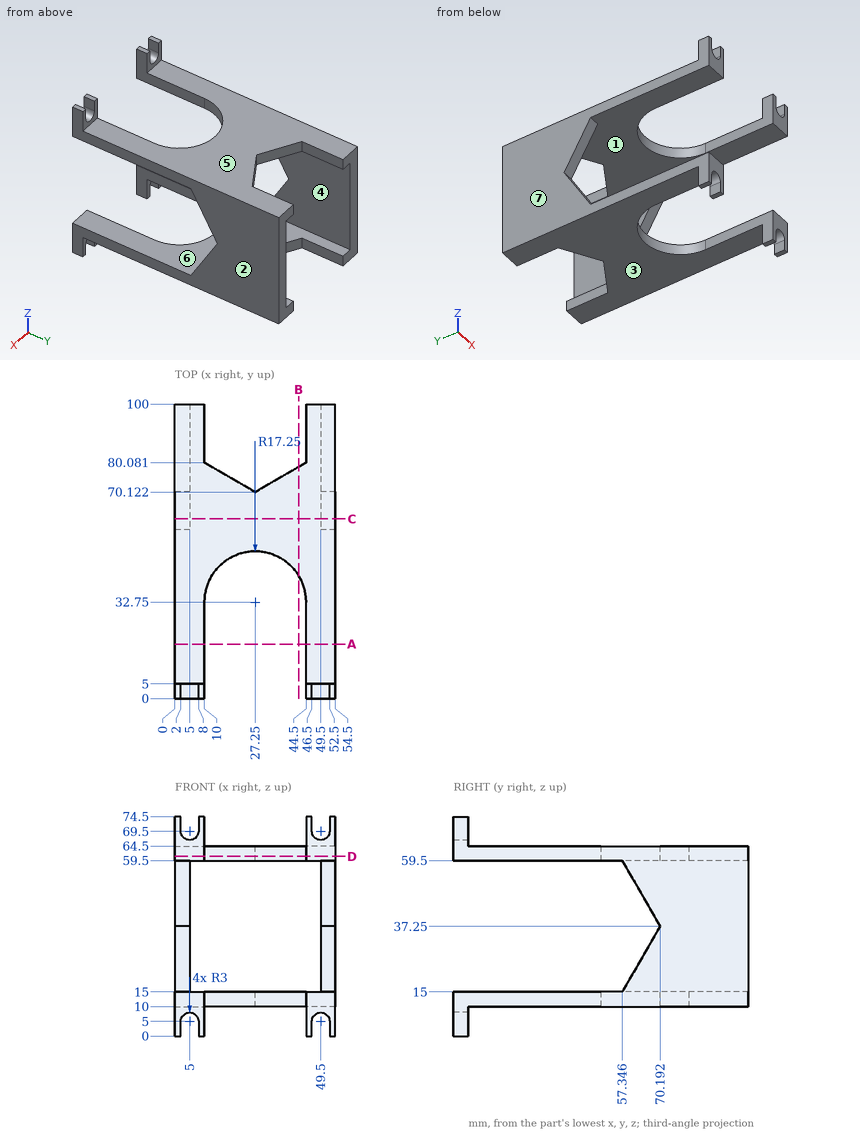
Input: dimensioned drawing with shaded views. Units: mm. Origin: part minimum x, y, z. A direction names the side the tool comes from. Coordinates: 2 decimals unless noted, no trailing zeros. Loops run counter-clockwise (first coordinate to the right, second up) from the corner with the lowest first, then second, coordinate; pieces in that order, holes last. Notation, with made-up numbers: M 39.5,-9 L 85.5,-9 A21 cw 85.5,27 Z; hole C 18,27 d4. An arc over 180 degrees is marked long. Put each result on its own line as item: value.
(1) Cut plane B-B on x = 42. Return the cut outline in (y, z) (1 decimal).
Answer sheet:
outline: M 41.7,10 L 78.6,10 L 78.6,15 L 41.7,15 Z; M 41.7,59.5 L 78.6,59.5 L 78.6,64.5 L 41.7,64.5 Z
(2) First-contact query: pin 1 (6 mm diameter, centred on x = 39, z = 59.5, fed in from +Y); pin 2 (11 mm diameter, centred on x = 5, z = 4, fed in from +Y); pin 3 (1.5 mm diameter, centred on y = 1.5, z = 72.5, fed in from -X); pin 4 (1.5 mm diameter, centred on x = 7, z = 54, fed in from -Y). Flat tips, straight axial feed; report the tip coordinate or a pass-through.
Answer sheet:
pin 1: stops at y = 78.64
pin 2: stops at y = 5
pin 3: stops at x = 0
pin 4: passes through
(3) Cut plane A-A on y = 18.5. Return the cut outline in (x, z), then the cut area to 3 significant figures.
Answer sheet:
outline: M 0,10 L 10,10 L 10,15 L 0,15 Z; M 0,59.5 L 10,59.5 L 10,64.5 L 0,64.5 Z; M 44.5,10 L 54.5,10 L 54.5,15 L 44.5,15 Z; M 44.5,59.5 L 54.5,59.5 L 54.5,64.5 L 44.5,64.5 Z
area: 200 mm^2
(4) Material intervals for probe 1 along X at (y, z) = (64, 54); probe 2 along Z at (x, y) = (52, 35); probe 3 along Z at (x, y) = (3, 89.5), sorted ascending.
Answer sheet:
probe 1: x = 0 to 5, 49.5 to 54.5
probe 2: z = 10 to 15, 59.5 to 64.5
probe 3: z = 10 to 64.5
(5) Cut plane C-C on y = 61. Return the cut outline in (x, z).
Answer sheet:
outline: M 0,10 L 54.5,10 L 54.5,21.33 L 49.5,21.33 L 49.5,15 L 5,15 L 5,21.33 L 0,21.33 Z; M 0,53.17 L 5,53.17 L 5,59.5 L 49.5,59.5 L 49.5,53.17 L 54.5,53.17 L 54.5,64.5 L 0,64.5 Z
(6) Cut plane D-D on z = 61. Return the cut outline in (x, y), then the cut area to 3 significant figures.
Answer sheet:
outline: M 0,0 L 10,0 L 10,32.75 A17.25 cw 44.5,32.75 L 44.5,0 L 54.5,0 L 54.5,100 L 44.5,100 L 44.5,80.08 L 27.25,70.12 L 10,80.08 L 10,100 L 0,100 Z
area: 2,990 mm^2
(7) Access query for the marked faces 1, 2, 3 and 4. Directions: +Z, -Z, +X, -X, +Y, -Y. A direction counts if a zero-diameter tool reaches every point of the face in a straight line with its end or side. Return the directions, or none.
Answer sheet:
face 1: -Y
face 2: +Z, -Z, +X, +Y, -Y
face 3: -Z, +X, -X, +Y
face 4: +Y, -Y
(8) Draft query along Z for the marked faces 5, 6 and 7. Return one class per face: pulls with the +Z half, pulls with the -Z half, needs draft (parallel to the pull), parting line crosses it, or undercut.
Answer sheet:
face 5: pulls with the +Z half
face 6: undercut
face 7: needs draft
